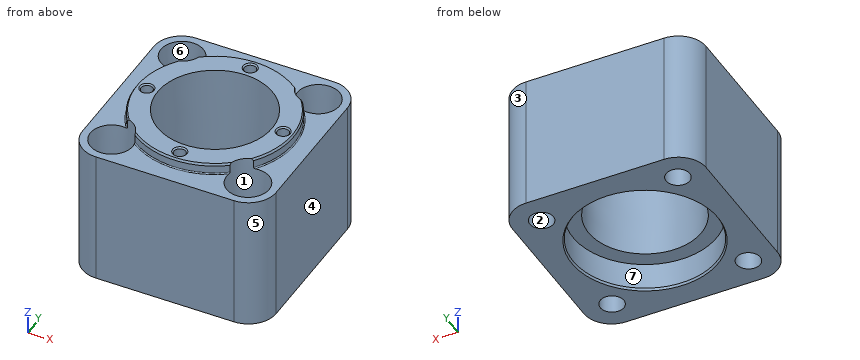
Autodesk Inventor part; units mm, degrees
ref_plane "ADAPTER_XY" through (0, 0, -38) normal (0, 0, 1) x (1, 0, 0)
ref_plane "ADAPTER_YZ" through (0, 0, -38) normal (1, 0, 0) x (0, 1, 0)
ref_plane "ADAPTER_ZX" through (0, 0, -38) normal (0, 1, 0) x (0, 0, 1)
sketch "Skizze_1" plane through (0, 0, -38) normal (0, 0, 1) x (1, 0, 0)
  line L0 (-27, 19.25) -> (-27, -19.25)
  arc A0 (-27, -19.25) -> (-19.25, -27) centre (-19.25, -19.25) ccw
  line L1 (-19.25, -27) -> (19.25, -27)
  arc A1 (19.25, -27) -> (27, -19.25) centre (19.25, -19.25) ccw
  line L2 (27, -19.25) -> (27, 19.25)
  arc A2 (27, 19.25) -> (19.25, 27) centre (19.25, 19.25) ccw
  line L3 (19.25, 27) -> (-19.25, 27)
  arc A3 (-19.25, 27) -> (-27, 19.25) centre (-19.25, 19.25) ccw
extrude "Extrusion1" add sketch "Skizze_1" along normal blind 38
sketch "Skizze_2" plane through (0, 0, 0) normal (1, 0, 0) x (0, 1, 0)
  line L0 (0, 0) -> (0, 3)
  line L1 (0, 3) -> (21.6536, 3)
  line L2 (21.6536, 3) -> (22, 2.4)
  line L3 (22, 2.4) -> (22, 0.3)
  arc A0 (22, 0.3) -> (22.3, 0) centre (22.3, 0.3) ccw
  line L4 (22.3, 0) -> (0, 0)
  line L5 (0, 0) -> (0, 3)
revolve "Revolution1" add sketch "Skizze_2" angle 360 about axis through (0, 0, 0) along (0, 0, 1)
sketch "Skizze_3" plane through (0, 0, 0) normal (1, 0, 0) x (0, 1, 0)
  line L0 (0, -38) -> (0, 3)
  line L1 (0, 3) -> (16, 3)
  line L2 (16, 3) -> (15.712, -30)
  line L3 (15.712, -30) -> (20, -30)
  line L4 (20, -30) -> (20, -37.4)
  line L5 (20, -37.4) -> (20.3464, -38)
  line L6 (20.3464, -38) -> (0, -38)
  line L7 (0, -38) -> (0, 3)
revolve "Revolution2" cut sketch "Skizze_3" angle 360 about axis through (0, 0, -38) along (0, 0, 1)
sketch "Sketch4" plane through (0, 0, 3) normal (0, 0, 1) x (1, 0, 0)
  point P0 (0, 19)
hole "Hole1" at (0, 19, 3) direction (0, 0, -1) diameter 3.242 depth 15 tip angle 120 countersink diameter 4 countersink angle 90
sketch "Sketch5" plane through (0, 0, 3) normal (0, 0, 1) x (1, 0, 0)
  point P0 (0, -19)
hole "Hole2" at (0, -19, 3) direction (0, 0, -1) diameter 3.242 depth 15 tip angle 120 countersink diameter 4 countersink angle 90
sketch "Sketch6" plane through (0, 0, 3) normal (0, 0, 1) x (1, 0, 0)
  point P0 (19, 0)
hole "Hole3" at (19, 0, 3) direction (0, 0, -1) diameter 3.242 depth 15 tip angle 120 countersink diameter 4 countersink angle 90
sketch "Sketch7" plane through (0, 0, 3) normal (0, 0, 1) x (1, 0, 0)
  point P0 (-19, 0)
hole "Hole4" at (-19, 0, 3) direction (0, 0, -1) diameter 3.242 depth 15 tip angle 120 countersink diameter 4 countersink angle 90
sketch "Skizze_8" plane through (19, 0, 0) normal (1, 0, 0) x (0, 0, -1)
  line L0 (38, 19) -> (-3, 19)
  line L1 (-3, 19) -> (-3, 24.9713)
  line L2 (-3, 24.9713) -> (24, 24.5)
  line L3 (24, 24.5) -> (24, 22.3)
  line L4 (24, 22.3) -> (38, 22.3)
  line L5 (38, 22.3) -> (38, 19)
  line L6 (38, 19) -> (-3, 19)
revolve "Revolution3" cut sketch "Skizze_8" angle 360 about axis through (19, 19, -38) along (0, 0, 1)
sketch "Skizze_9" plane through (19, 0, 0) normal (1, 0, 0) x (0, 0, -1)
  line L0 (38, -19) -> (-3, -19)
  line L1 (-3, -19) -> (-3, -13.0287)
  line L2 (-3, -13.0287) -> (24, -13.5)
  line L3 (24, -13.5) -> (24, -15.7)
  line L4 (24, -15.7) -> (38, -15.7)
  line L5 (38, -15.7) -> (38, -19)
  line L6 (38, -19) -> (-3, -19)
revolve "Revolution4" cut sketch "Skizze_9" angle 360 about axis through (19, -19, -38) along (0, 0, 1)
sketch "Skizze_10" plane through (-19, 0, 0) normal (1, 0, 0) x (0, 0, -1)
  line L0 (38, 19) -> (-3, 19)
  line L1 (-3, 19) -> (-3, 24.9713)
  line L2 (-3, 24.9713) -> (24, 24.5)
  line L3 (24, 24.5) -> (24, 22.3)
  line L4 (24, 22.3) -> (38, 22.3)
  line L5 (38, 22.3) -> (38, 19)
  line L6 (38, 19) -> (-3, 19)
revolve "Revolution5" cut sketch "Skizze_10" angle 360 about axis through (-19, 19, -38) along (0, 0, 1)
sketch "Skizze_11" plane through (-19, 0, 0) normal (1, 0, 0) x (0, 0, -1)
  line L0 (38, -19) -> (-3, -19)
  line L1 (-3, -19) -> (-3, -13.0287)
  line L2 (-3, -13.0287) -> (24, -13.5)
  line L3 (24, -13.5) -> (24, -15.7)
  line L4 (24, -15.7) -> (38, -15.7)
  line L5 (38, -15.7) -> (38, -19)
  line L6 (38, -19) -> (-3, -19)
revolve "Revolution6" cut sketch "Skizze_11" angle 360 about axis through (-19, -19, -38) along (0, 0, 1)
ref_plane "ADAPTER_XY" through (0, 0, -38) normal (0, 0, 1) x (1, 0, 0)
ref_plane "ADAPTER_YZ" through (0, 0, -38) normal (1, 0, 0) x (0, 1, 0)
ref_plane "ADAPTER_ZX" through (0, 0, -38) normal (0, 1, 0) x (0, 0, 1)
ref_plane "ANBAU_XY" through (0, 0, -38) normal (0, 0, 1) x (1, 0, 0)
ref_plane "ANBAU_YZ" through (0, 0, -38) normal (1, 0, 0) x (0, 1, 0)
ref_plane "ANBAU_ZX" through (0, 0, -38) normal (0, 1, 0) x (0, 0, 1)
ref_plane "ANBAU_1_XY" through (0, 0, 3) normal (0, 0, 1) x (1, 0, 0)
ref_plane "ANBAU_1_YZ" through (0, 0, 3) normal (1, 0, 0) x (0, 1, 0)
ref_plane "ANBAU_1_ZX" through (0, 0, 3) normal (0, 1, 0) x (0, 0, 1)
ref_plane "EAMK_XY" through (0, 0, -38) normal (0, 0, 1) x (1, 0, 0)
ref_plane "EAMK_YZ" through (0, 0, -38) normal (1, 0, 0) x (0, 1, 0)
ref_plane "EAMK_ZX" through (0, 0, -38) normal (0, 1, 0) x (0, 0, 1)
ref_plane "Kupplung_XY" through (0, 0, -29.6) normal (0, 0, -1) x (1, 0, 0)
ref_plane "Kupplung_YZ" through (0, 0, -29.6) normal (1, 0, 0) x (0, -1, 0)
ref_plane "Kupplung_ZX" through (0, 0, -29.6) normal (0, -1, 0) x (0, 0, -1)
ref_plane "MOTORFLANSCH_XY" through (0, 0, 0) normal (0, 0, 1) x (1, 0, 0)
ref_plane "MOTORFLANSCH_YZ" through (0, 0, 0) normal (1, 0, 0) x (0, 1, 0)
ref_plane "MOTORFLANSCH_ZX" through (0, 0, 0) normal (0, 1, 0) x (0, 0, 1)
ref_plane "ZYL_SCHRAUBE_1_1_XY" through (-19, 19, -24) normal (0, 0, 1) x (1, 0, 0)
ref_plane "ZYL_SCHRAUBE_1_1_YZ" through (-19, 19, -24) normal (1, 0, 0) x (0, 1, 0)
ref_plane "ZYL_SCHRAUBE_1_1_ZX" through (-19, 19, -24) normal (0, 1, 0) x (0, 0, 1)
ref_plane "ZYL_SCHRAUBE_1_2_XY" through (19, 19, -24) normal (0, 0, 1) x (1, 0, 0)
ref_plane "ZYL_SCHRAUBE_1_2_YZ" through (19, 19, -24) normal (1, 0, 0) x (0, 1, 0)
ref_plane "ZYL_SCHRAUBE_1_2_ZX" through (19, 19, -24) normal (0, 1, 0) x (0, 0, 1)
ref_plane "ZYL_SCHRAUBE_1_3_XY" through (19, -19, -24) normal (0, 0, 1) x (1, 0, 0)
ref_plane "ZYL_SCHRAUBE_1_3_YZ" through (19, -19, -24) normal (1, 0, 0) x (0, 1, 0)
ref_plane "ZYL_SCHRAUBE_1_3_ZX" through (19, -19, -24) normal (0, 1, 0) x (0, 0, 1)
ref_plane "ZYL_SCHRAUBE_1_4_XY" through (-19, -19, -24) normal (0, 0, 1) x (1, 0, 0)
ref_plane "ZYL_SCHRAUBE_1_4_YZ" through (-19, -19, -24) normal (1, 0, 0) x (0, 1, 0)
ref_plane "ZYL_SCHRAUBE_1_4_ZX" through (-19, -19, -24) normal (0, 1, 0) x (0, 0, 1)
ref_plane "ZYL_SCHRAUBE_2_1_XY" through (22.2739, 22.2739, 0) normal (0, 0, 1) x (1, 0, 0)
ref_plane "ZYL_SCHRAUBE_2_1_YZ" through (22.2739, 22.2739, 0) normal (1, 0, 0) x (0, 1, 0)
ref_plane "ZYL_SCHRAUBE_2_1_ZX" through (22.2739, 22.2739, 0) normal (0, 1, 0) x (0, 0, 1)
ref_plane "ZYL_SCHRAUBE_2_2_XY" through (-22.2739, 22.2739, 0) normal (0, 0, 1) x (1, 0, 0)
ref_plane "ZYL_SCHRAUBE_2_2_YZ" through (-22.2739, 22.2739, 0) normal (1, 0, 0) x (0, 1, 0)
ref_plane "ZYL_SCHRAUBE_2_2_ZX" through (-22.2739, 22.2739, 0) normal (0, 1, 0) x (0, 0, 1)
ref_plane "ZYL_SCHRAUBE_2_3_XY" through (-22.2739, -22.2739, 0) normal (0, 0, 1) x (1, 0, 0)
ref_plane "ZYL_SCHRAUBE_2_3_YZ" through (-22.2739, -22.2739, 0) normal (1, 0, 0) x (0, 1, 0)
ref_plane "ZYL_SCHRAUBE_2_3_ZX" through (-22.2739, -22.2739, 0) normal (0, 1, 0) x (0, 0, 1)
ref_plane "ZYL_SCHRAUBE_2_4_XY" through (22.2739, -22.2739, 0) normal (0, 0, 1) x (1, 0, 0)
ref_plane "ZYL_SCHRAUBE_2_4_YZ" through (22.2739, -22.2739, 0) normal (1, 0, 0) x (0, 1, 0)
ref_plane "ZYL_SCHRAUBE_2_4_ZX" through (22.2739, -22.2739, 0) normal (0, 1, 0) x (0, 0, 1)
ref_plane "ZYL_SCHRAUBE_2x_1_XY" through (23.57, 23.57, 0) normal (0, 0, 1) x (1, 0, 0)
ref_plane "ZYL_SCHRAUBE_2x_1_YZ" through (23.57, 23.57, 0) normal (1, 0, 0) x (0, 1, 0)
ref_plane "ZYL_SCHRAUBE_2x_1_ZX" through (23.57, 23.57, 0) normal (0, 1, 0) x (0, 0, 1)
ref_plane "ZYL_SCHRAUBE_2x_2_XY" through (-23.57, 23.57, 0) normal (0, 0, 1) x (1, 0, 0)
ref_plane "ZYL_SCHRAUBE_2x_2_YZ" through (-23.57, 23.57, 0) normal (1, 0, 0) x (0, 1, 0)
ref_plane "ZYL_SCHRAUBE_2x_2_ZX" through (-23.57, 23.57, 0) normal (0, 1, 0) x (0, 0, 1)
ref_plane "ZYL_SCHRAUBE_2x_3_XY" through (-23.57, -23.57, 0) normal (0, 0, 1) x (1, 0, 0)
ref_plane "ZYL_SCHRAUBE_2x_3_YZ" through (-23.57, -23.57, 0) normal (1, 0, 0) x (0, 1, 0)
ref_plane "ZYL_SCHRAUBE_2x_3_ZX" through (-23.57, -23.57, 0) normal (0, 1, 0) x (0, 0, 1)
ref_plane "ZYL_SCHRAUBE_2x_4_XY" through (23.57, -23.57, 0) normal (0, 0, 1) x (1, 0, 0)
ref_plane "ZYL_SCHRAUBE_2x_4_YZ" through (23.57, -23.57, 0) normal (1, 0, 0) x (0, 1, 0)
ref_plane "ZYL_SCHRAUBE_2x_4_ZX" through (23.57, -23.57, 0) normal (0, 1, 0) x (0, 0, 1)
ref_plane "ZYL_SCHRAUBE_3_1_XY" through (19, 0, 4.7) normal (0, 0, 1) x (1, 0, 0)
ref_plane "ZYL_SCHRAUBE_3_1_YZ" through (19, 0, 4.7) normal (1, 0, 0) x (0, 1, 0)
ref_plane "ZYL_SCHRAUBE_3_1_ZX" through (19, 0, 4.7) normal (0, 1, 0) x (0, 0, 1)
ref_plane "ZYL_SCHRAUBE_3_2_XY" through (0, -19, 4.7) normal (0, 0, 1) x (1, 0, 0)
ref_plane "ZYL_SCHRAUBE_3_2_YZ" through (0, -19, 4.7) normal (1, 0, 0) x (0, 1, 0)
ref_plane "ZYL_SCHRAUBE_3_2_ZX" through (0, -19, 4.7) normal (0, 1, 0) x (0, 0, 1)
ref_plane "ZYL_SCHRAUBE_3_3_XY" through (-19, 0, 4.7) normal (0, 0, 1) x (1, 0, 0)
ref_plane "ZYL_SCHRAUBE_3_3_YZ" through (-19, 0, 4.7) normal (1, 0, 0) x (0, 1, 0)
ref_plane "ZYL_SCHRAUBE_3_3_ZX" through (-19, 0, 4.7) normal (0, 1, 0) x (0, 0, 1)
ref_plane "to_eamf_XY" through (0, 0, 0.5) normal (0, 0, 1) x (1, 0, 0)
ref_plane "to_eamf_YZ" through (0, 0, 0.5) normal (1, 0, 0) x (0, 1, 0)
ref_plane "to_eamf_ZX" through (0, 0, 0.5) normal (0, 1, 0) x (0, 0, 1)
properties part number "552157 EAMK-A-D40-44A/C---(1O)"
Here's how the part is built. I have some questions about the finished solid (model axes, mm). Face numbers are marked on the shaded views. A direction names the side the tool comes from. Round coordinates to 2 decimals unless told otherwise and drop trailing zeros. Order: outer loops, then holes, each group sorted by start corner. A loop starts at its lowest first (then second) coordinate and runs counter-clockwise, first axis right, second up. Notation, with made-up numbers: (-27.5, 80.25) -> (16.5, 80.25) arc R19 cw to (16.5, 92.25) -> close; hole circle Ø1 at (-37, 76). An arc over 180 degrees is marked (long way). Return JSON: item names as keys, results as strings.
Q1. Which directions (+Z, -Z, +X, -X, +Y, -Y) give clear straight access to the entire face, cutting with the end or side of a thin tool? Please do the marked faces 5, 6 and 7.
Filled sheet:
{"face 5": "+Z, -Z, +X, -Y", "face 6": "+Z", "face 7": "-Z"}
Q2. For pin 1 Ø6 at (x, y) = (11, 10) entering from -Z; pin 2 Ø5.5 at (x, y) = (-20.5, 17.5) entering from +Z; pin 3 Ø2 at (x, z) = (21.5, -30.5) entering from -Y, each with a flat end and sliding along its axis, tell me the tip position at first contact or that it passes through.
Filled sheet:
{"pin 1": "stops at z = -30", "pin 2": "stops at z = -24", "pin 3": "stops at y = -26.9"}
Q3. If we section it at A-A on z = -11: Give the number of separate pieces and of enclosed holes in the cut face, plus the area to 3 significant figures.
Filled sheet:
{"separate pieces": "1", "enclosed holes": "9", "area": "1,630 mm^2"}
Q4. If we section it at B-B on z = -26: List the corners of the cut face in (x, y) for me, plus the area to 3 significant figures.
Filled sheet:
{"outline": "(-27, -19.25) arc R7.75 ccw to (-19.25, -27) -> (19.25, -27) arc R7.75 ccw to (27, -19.25) -> (27, 19.25) arc R7.75 ccw to (19.25, 27) -> (-19.25, 27) arc R7.75 ccw to (-27, 19.25) -> close; hole circle Ø6.6 at (-19, -19); hole circle Ø6.6 at (-19, 19); hole circle Ø31.49 at (0, 0); hole circle Ø6.6 at (19, -19); hole circle Ø6.6 at (19, 19)", "area": "1,950 mm^2"}
Q5. If we mould it in two halves opening along Y, with no side actions, what happens to the marked faces 1, 2, 3 and 4? For each: released by +Y, released by -Y, zero draft, split by the parting line, or undercut.
Filled sheet:
{"face 1": "undercut", "face 2": "undercut", "face 3": "released by +Y", "face 4": "zero draft"}
Q6. I need wall thicknesses on line 1 along Y through (x, z) = (-17.5, -13); line 2 along Y through (x, z) = (19, -28); line 3 along Y through (x, z) = (0, -31.5). Which ranges of each line are inside material? Lowest first, please. Write a range as from..to.
Filled sheet:
{"line 1": "y = -27..-24.49, -13.51..13.51, 24.49..27", "line 2": "y = -27..-22.3, -15.7..15.7, 22.3..27", "line 3": "y = -27..-20, 20..27"}
